Part print with two shaded views. Sizes in mm from the minimum x, y, z corner. Round coordinates to 2 decimals unless told otherwise and drop trailing zeros. Loops run counter-clockwise (first coordinate to the right, second up) from the corner with the lowest first, then second, coordinate; pieces in that order, holes last.
(1) Cut at C-C on y = 94.5. List the corners of the cut face in (x, z), then the cut area to 3 significant figures.
(2) Cut at B-B on x = 76.2. List the corners of the cut face in (y, z).
(3) Cut at A-A on x = 133.35. List the corners of the cut face in (y, z), then the cut area to 3 significant figures.
(4) Probe probe 1 along Y at (x, z) = (19.05, 1.95); probe 2 along Y at (x, z) = (76.2, 1.15); probe 3 along X at (y, z) = (88.9, 1). List the from-to ranges inside material, lowest first.
(5) Flat gauge pin, fed straight in: pin 1 (11.5 mm diameter, centred on x = 133.35, y = 17.399, fed in from -Z). Where does the tip first touch, or does it go through?
(6) Cut at D-D on z = 0.4. List the corners of the cut face in (x, y), then the cut area to 3 significant figures.
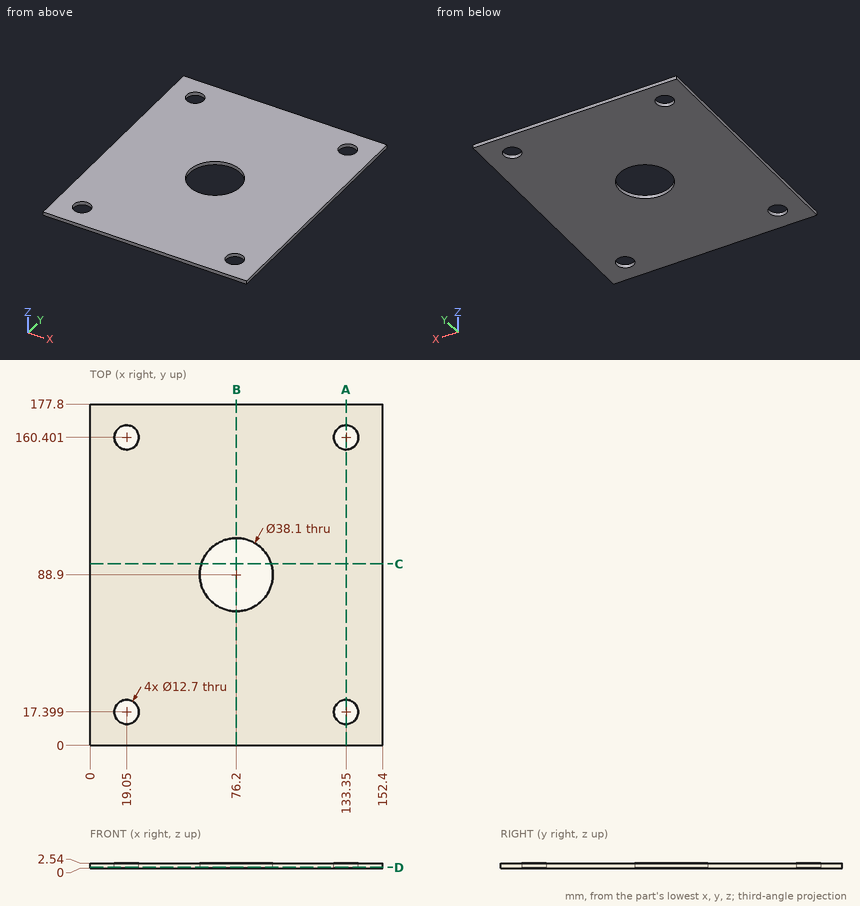
Final values:
1. outline: (0, 0) - (57.99, 0) - (57.99, 2.54) - (0, 2.54) - close; (94.41, 0) - (152.4, 0) - (152.4, 2.54) - (94.41, 2.54) - close
1. area: 295 mm2
2. outline: (0, 0) - (69.85, 0) - (69.85, 2.54) - (0, 2.54) - close; (107.95, 0) - (177.8, 0) - (177.8, 2.54) - (107.95, 2.54) - close
3. outline: (0, 0) - (11.05, 0) - (11.05, 2.54) - (0, 2.54) - close; (23.75, 0) - (154.05, 0) - (154.05, 2.54) - (23.75, 2.54) - close; (166.75, 0) - (177.8, 0) - (177.8, 2.54) - (166.75, 2.54) - close
3. area: 387 mm2
4. probe 1: y = 0 to 11.05, 23.75 to 154.05, 166.75 to 177.8
4. probe 2: y = 0 to 69.85, 107.95 to 177.8
4. probe 3: x = 0 to 57.15, 95.25 to 152.4
5. pin 1: passes through
6. outline: (0, 0) - (152.4, 0) - (152.4, 177.8) - (0, 177.8) - close; hole circle Ø12.7 at (19.05, 17.4); hole circle Ø12.7 at (19.05, 160.4); hole circle Ø38.1 at (76.2, 88.9); hole circle Ø12.7 at (133.35, 17.4); hole circle Ø12.7 at (133.35, 160.4)
6. area: 25,400 mm2
